Solid Edge part; units mm, degrees
sketch "Sketch1" plane through (0, 0, 0) normal (0, 0, 1) x (1, 0, 0)
  line L0 (2.5, 0) -> (2.5, 8)
  line L1 (0, 8) -> (2.5, 8)
  line L2 (0, 0) -> (0, 8)
  line L3 (0, 0) -> (0, -5)
  line L4 (0, -5) -> (4.25, -5)
  line L5 (4.25, -5) -> (4.25, 0)
  line L6 (4.25, 0) -> (2.5, 0)
revolve "RevolvedProtrusion1" add sketch "Sketch1" angle 360 about axis through (0, 0, 0) along (0, 1, 0)
sketch "Sketch2" plane through (0, 0, 0) normal (1, 0, 0) x (0, 1, 0)
  line L0 (-5, 2.7915) -> (-2.5, 2.7915)
  line L1 (-0.8883, 0) -> (-2.5, 2.7915)
  line L2 (-5, 0) -> (-0.8883, 0)
  line L3 (-5, 0) -> (-5, 2.7915)
revolve "RevolvedCutout1" cut sketch "Sketch2" angle 360 about axis through (0, -4.5, 0) along (0, 1, 0)
sketch "Sketch3" plane through (0, -5, 0) normal (0, -1, 0) x (0, 0, 1)
  circle A0 centre (0, 0) radius 2.7915
  line L0 (-2, -1.1547) -> (0, -2.3094)
  line L1 (0, -2.3094) -> (2, -1.1547)
  line L2 (2, -1.1547) -> (2, 1.1547)
  line L3 (2, 1.1547) -> (0, 2.3094)
  line L4 (0, 2.3094) -> (-2, 1.1547)
  line L5 (-2, 1.1547) -> (-2, -1.1547)
extrude "Protrusion1" add sketch "Sketch3" against normal up to next
sketch "Sketch4" plane through (0, 0, 0) normal (0, 0, 1) x (1, 0, 0)
  line L0 (-2.3094, -5) -> (0, -5)
  line L1 (0, -5) -> (0, -4.3812)
  line L2 (0, -4.3812) -> (-2.3094, -5)
revolve "RevolvedCutout2" cut sketch "Sketch4" angle 360 about axis through (0, -4.5, 0) along (0, 1, 0)
fillet "Round1" radius 0.2 1 edges at (0, 0, -2.5)
fillet "Round2" radius 0.425 1 edges at (0, -5, -4.25)
chamfer "倒斜角_2" distance 0.3333 angle 45 1 edges at (0, 8, -2.5)
cosmetic_thread "螺纹_3" thread depth 6.4
The listing builds one solid part. Answer for the finished solid, in the listing's coordinates (mm). A direction names the side the tool comes from. Give positions to 0.01 mm unless a question says otherwise; leave off trailing zeros. Loops run counter-clockwise (first coordinate to the right, second up) from the corner with the lowest first, then second, coordinate; pieces in that order, holes last. Notation, with made-up numbers: (4, 56) - (54, 56) arc R20 cw to (54, 67) - close; hole circle Ø10 at (50.5, 38.5). An arc over 180 degrees is marked (long way). Answer as CSV lines item,"result". Start each with the question number.
Item 1: For faces 1 (the face through (0, 8, 0)), 2 (the face through (-0.54, 3.99, 2.44)), 3 (the face through (1.88, -4.96, 1.06)), determine the directions among +Z, -Z, +X, -X, +Y, -Y from which every point of the face is accessible in a straight line to the end or side of a thin tool.
Item 2: A cutting plane is placed at C-C on y = -0.25. Determine the outline of the cut face in (x, z), then the cut area to 3 significant figures.
Item 3: A cutting plane is placed at A-A on y = -4. Determine the outline of the cut face in (x, z).
Item 4: Find the intervals of material crossed by line 1 (Y direction, x = -3.5, z = 0); line 2 (X direction, y = 3, z = -1.5); line 3 (Z direction, x = 2, y = 1.75), in increasing order. Write a range as from..to.
Item 5: The mould has two halves that part along X. Classify faces 4 (the face through (2, -5, 2)), 5 (the face through (-1.88, -4.96, -1.06)), 6 (the face through (2.285, -2.255, -3.584)): +X half, -X half, draft (parallel to the pull), parting line (faces both ways), or undercut.
Item 6: A cutting plane is placed at B-B on y = 4.75. Determine the outline of the cut face in (x, z), then the cut area to 3 significant figures.
Item 7: Each of these flat-tipped pins is pushed along its axis until it touches: pin 1 (3 mm diameter, centred on x = 2, y = 4.5, fed in from -Z); pin 2 (2 mm diameter, centred on y = 1.5, z = -0.5, fed in from -X). Where does it stop, or does it pass through?
Found:
1,face 1,"+Z, -Z, +X, -X, +Y"
1,face 2,"+Y"
1,face 3,"-Y"
2,outline,"circle Ø8.5 at (0, 0)"
2,area,"56.7 mm^2"
3,outline,"circle Ø8.5 at (0, 0); hole (-2.31, 0) - (-1.15, -2) - (1.15, -2) - (2.31, 0) - (1.15, 2) - (-1.15, 2) - close"
4,line 1,"y = -5..0"
4,line 2,"x = -2..2"
4,line 3,"z = -1.5..1.5"
5,face 4,"draft"
5,face 5,"undercut"
5,face 6,"parting line"
6,outline,"circle Ø5 at (0, 0)"
6,area,"19.6 mm^2"
7,pin 1,"stops at z = -2.45"
7,pin 2,"stops at x = -2.5"
